Could you check a few things on this model? Use its own coordinates, in mm. A direction names the side the tool comes from. Round coordinates to 2 decimals unless told otherwise and drop trailing zeros. Loops run counter-clockwise (first coordinate to the right, second up) from the corner with the lowest first, then second, coordinate; pieces in that order, holes last. Notation, with made-up numbers: M 42,-23 L 52,-23 A12 cw 52,-5 Z; hole C -16,-20 d2. An arc over 180 degrees is marked long. Answer in a Markdown table with one row per item.
```python
from build123d import *

# Parameters (mm, degrees)
F0_R     = 9.525
F1_DEPTH = 3.175


with BuildPart() as f1:
    # F0 (on Front) → F1 (new body)
    with BuildSketch(Plane.XZ):
        with BuildLine():
            ThreePointArc((41.275, 0), (29.1858323935, 29.1858323935), (0, 41.275))
            ThreePointArc((0, 41.275), (-29.1858323935, -29.1858323935), (41.275, 0))
        make_face()
        with BuildLine():
            ThreePointArc((26.9407683632, 26.9407683632), (35.1998101887, 14.5802387731), (38.1, 0))
            ThreePointArc((38.1, 0), (35.1998101887, -14.5802387731), (26.9407683632, -26.9407683632))
            ThreePointArc((26.9407683632, -26.9407683632), (14.5802387731, -35.1998101887), (0, -38.1))
            ThreePointArc((0, -38.1), (-14.5802387731, -35.1998101887), (-26.9407683632, -26.9407683632))
            ThreePointArc((-26.9407683632, -26.9407683632), (-35.1998101887, -14.5802387731), (-38.1, 0))
            ThreePointArc((-38.1, 0), (-35.1998101887, 14.5802387731), (-26.9407683632, 26.9407683632))
            ThreePointArc((-26.9407683632, 26.9407683632), (-14.5802387731, 35.1998101887), (0, 38.1))
            ThreePointArc((0, 38.1), (14.5802387731, 35.1998101887), (26.9407683632, 26.9407683632))
        make_face(mode=Mode.SUBTRACT)
        with BuildLine():
            ThreePointArc((26.9407683632, -26.9407683632), (35.1998101887, -14.5802387731), (38.1, 0))
            Line((38.1, 0), (12.7, 0))
            ThreePointArc((12.7, 0), (11.7332700629, -4.860079591), (8.9802561211, -8.9802561211))
            Line((8.9802561211, -8.9802561211), (26.9407683632, -26.9407683632))
        make_face()
        with BuildLine():
            Line((8.9802561211, 8.9802561211), (26.9407683632, 26.9407683632))
            ThreePointArc((26.9407683632, 26.9407683632), (14.5802387731, 35.1998101887), (0, 38.1))
            Line((0, 38.1), (0, 12.7))
            ThreePointArc((0, 12.7), (4.860079591, 11.7332700629), (8.9802561211, 8.9802561211))
        make_face()
        with BuildLine():
            ThreePointArc((8.9802561211, -8.9802561211), (11.7332700629, -4.860079591), (12.7, 0))
            ThreePointArc((12.7, 0), (11.7332700629, 4.860079591), (8.9802561211, 8.9802561211))
            ThreePointArc((8.9802561211, 8.9802561211), (4.860079591, 11.7332700629), (0, 12.7))
            ThreePointArc((0, 12.7), (-4.860079591, 11.7332700629), (-8.9802561211, 8.9802561211))
            ThreePointArc((-8.9802561211, 8.9802561211), (-11.7332700629, 4.860079591), (-12.7, 0))
            ThreePointArc((-12.7, 0), (-11.7332700629, -4.860079591), (-8.9802561211, -8.9802561211))
            ThreePointArc((-8.9802561211, -8.9802561211), (-4.860079591, -11.7332700629), (0, -12.7))
            ThreePointArc((0, -12.7), (4.860079591, -11.7332700629), (8.9802561211, -8.9802561211))
        make_face()
        Circle(F0_R, mode=Mode.SUBTRACT)
        with BuildLine():
            ThreePointArc((-26.9407683632, -26.9407683632), (-14.5802387731, -35.1998101887), (0, -38.1))
            Line((0, -38.1), (0, -12.7))
            ThreePointArc((0, -12.7), (-4.860079591, -11.7332700629), (-8.9802561211, -8.9802561211))
            Line((-8.9802561211, -8.9802561211), (-26.9407683632, -26.9407683632))
        make_face()
        with BuildLine():
            Line((-8.9802561211, 8.9802561211), (-26.9407683632, 26.9407683632))
            ThreePointArc((-26.9407683632, 26.9407683632), (-35.1998101887, 14.5802387731), (-38.1, 0))
            Line((-38.1, 0), (-12.7, 0))
            ThreePointArc((-12.7, 0), (-11.7332700629, 4.860079591), (-8.9802561211, 8.9802561211))
        make_face()
        Circle(F0_R)
    extrude(amount=F1_DEPTH)


solid = f1.part
```
1) Which directions (+Z, -Z, +X, -X, +Y, -Y) give clear straight access to the entire face, cutting with the end or side of a thin tool? Please do faces 1 (the face through (-1, 0, 1)), 2 (the face through (11.76, -1.57, 4.8)).
Computed:
| item | result |
|---|---|
| face 1 | +Z, -Z, +X, -X, +Y |
| face 2 | +Y, -Y |
2) Will these pins go through, and if not, where does the flat tip stop? P1, Ø5, axis at x = 22.5, z = 4, coming from the +Y side; P2, Ø1.6, axis at x = -23, y = -1, coming from the -Z side.
Computed:
| item | result |
|---|---|
| P1 | passes through |
| P2 | stops at z = -34.8 |
3) I need wall thicknesses on line 1 (X direction, y = -1.7, z = 19.5); line 2 (Z direction, x = 0.5, y = -2.15); line 3 (Z direction, x = -18, y = -1.6). Which ranges of each line are inside material? Lowest first, please.
Computed:
| item | result |
|---|---|
| line 1 | x = -36.38 to -19.5, 0 to 19.5, 32.73 to 36.38 |
| line 2 | z = -41.27 to -38.1, -12.69 to 41.27 |
| line 3 | z = -37.14 to -18, 0 to 18, 33.58 to 37.14 |
4) I want a section at A-A, the plane y = -1.45. Please give me the cut outline in (x, z) (3 decimals).
Computed:
| item | result |
|---|---|
| outline | C 0,0 d82.55; hole M -38.1,0 A38.1 ccw -26.941,-26.941 L -8.98,-8.98 A12.7 cw -12.7,0 Z; hole M -26.941,26.941 L -8.98,8.98 A12.7 cw 0,12.7 L 0,38.1 A38.1 ccw Z; hole M 0,-38.1 A38.1 ccw 26.941,-26.941 L 8.98,-8.98 A12.7 cw 0,-12.7 Z; hole M 8.98,8.98 A12.7 cw 12.7,0 L 38.1,0 A38.1 ccw 26.941,26.941 Z |
5) If we mould it in two halves opening along Z, with no side actions, what happens to faces 3 (the face through (-1, -3.175, 1)), 4 (the face through (14.77, -1.57, -35.12))? For each: released by +Z, released by -Z, zero draft, split by the parting line, or undercut.
Computed:
| item | result |
|---|---|
| face 3 | zero draft |
| face 4 | undercut |
6) I want a section at D-D, the plane z = -7. Please give me the cut outline in (x, y) (3 decimals), plus the area to 3 significant figures.
Computed:
| item | result |
|---|---|
| outline | M -40.677,-3.175 L -37.451,-3.175 L -37.451,0 L -40.677,0 Z; M -10.597,-3.175 L 40.677,-3.175 L 40.677,0 L -10.597,0 Z |
| area | 173 mm² |
7) I want a section at C-C, the plane x = -19.5. Please give me the cut outline in (y, z) (3 decimals), plus the area to 3 significant figures.
Computed:
| item | result |
|---|---|
| outline | M -3.175,-36.378 L 0,-36.378 L 0,-19.5 L -3.175,-19.5 Z; M -3.175,0 L 0,0 L 0,19.5 L -3.175,19.5 Z; M -3.175,32.732 L 0,32.732 L 0,36.378 L -3.175,36.378 Z |
| area | 127 mm² |
8) I want a section at B-B, the plane z = 14. Please give me the cut outline in (x, y) (3 decimals).
Computed:
| item | result |
|---|---|
| outline | M -38.828,-3.175 L -14,-3.175 L -14,0 L -38.828,0 Z; M 0,-3.175 L 14,-3.175 L 14,0 L 0,0 Z; M 35.435,-3.175 L 38.828,-3.175 L 38.828,0 L 35.435,0 Z |
